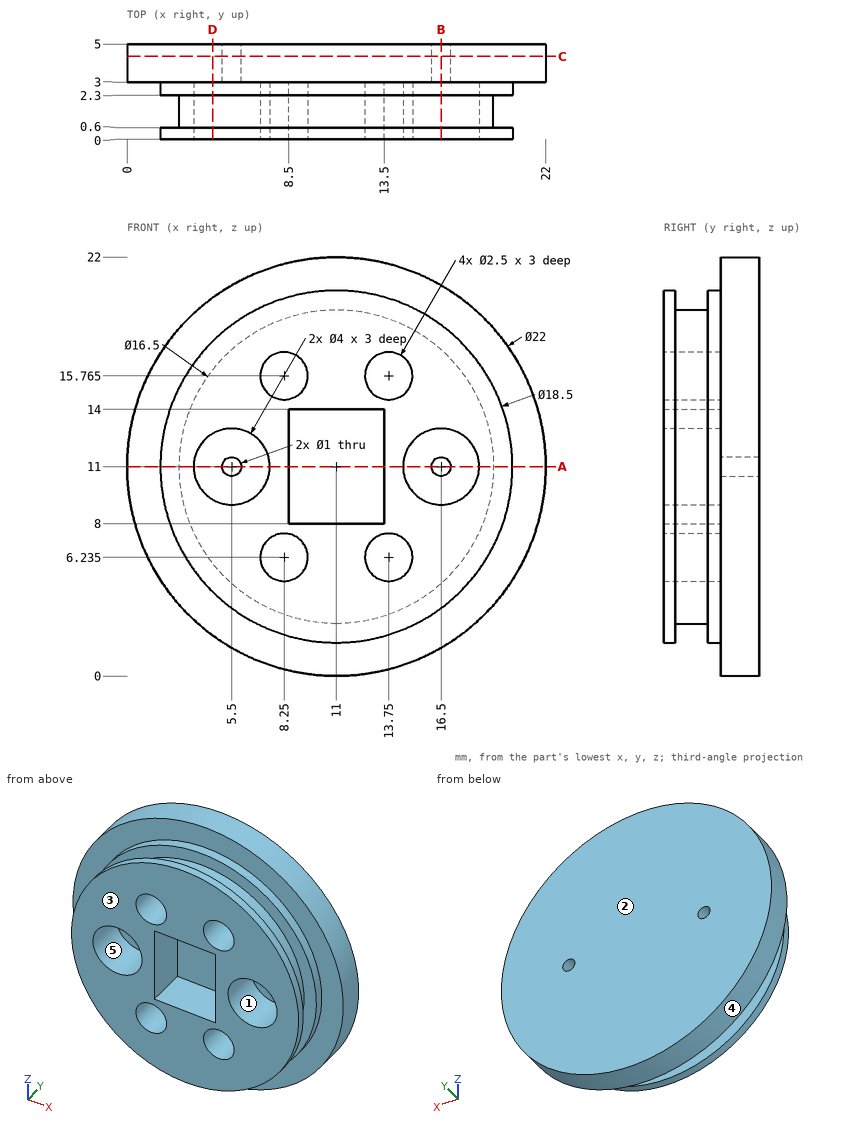
For this review, use the dimensioned drawing (mm, ordinates from the lowest corner) and the shaded views. A direction names the side the tool comes from. Coordinates: 2 decimals unless noted, no trailing zeros. Loops run counter-clockwise (first coordinate to the right, second up) from the corner with the lowest first, then second, coordinate; pieces in that order, holes last. Notation, with made-up numbers: (11.25, 23) -> (34.25, 23) arc R34 cw to (34.25, 54) -> close; hole circle Ø8 at (11.5, 46). An arc over 180 degrees is marked (long way). Write each question's results on one line, items separated by ' | '.
Q1. Mouldability with a two-part tool opening along Z and no side actions: class the marked faces 3, 4 and 5 as +Z half, -Z half, draft (parallel to the pull), parting line (faces both ways), or undercut.
Taken from the geometry:
face 3: draft | face 4: parting line | face 5: undercut
Q2. Machinability: for the marked faces 1 and 2, which of the approach directions +Z, -Z, +X, -X, +Y, -Y give a long, thin tool a straight path to every point of the face, cutting with its end or side? Answer none if there is none.
Taken from the geometry:
face 1: -Y | face 2: +Z, -Z, +X, -X, +Y
Q3. Add section B-B, the plane x = 16.5. State the section outline as (y, z) points, then the cut area to 3 significant figures.
Taken from the geometry:
outline: (0, 3.56) -> (0.6, 3.56) -> (0.6, 4.85) -> (2.3, 4.85) -> (2.3, 3.56) -> (3, 3.56) -> (3, 1.47) -> (5, 1.47) -> (5, 10.5) -> (3, 10.5) -> (3, 9) -> (0, 9) -> close; (0, 13) -> (3, 13) -> (3, 11.5) -> (5, 11.5) -> (5, 20.53) -> (3, 20.53) -> (3, 18.44) -> (2.3, 18.44) -> (2.3, 17.15) -> (0.6, 17.15) -> (0.6, 18.44) -> (0, 18.44) -> close | area: 64.3 mm²
Q4. Add section D-D, the plane x = 4.5. State the section outline as (y, z) points, then the cut area to 3 significant figures.
Taken from the geometry:
outline: (0, 4.42) -> (0.6, 4.42) -> (0.6, 5.92) -> (2.3, 5.92) -> (2.3, 4.42) -> (3, 4.42) -> (3, 2.13) -> (5, 2.13) -> (5, 19.87) -> (3, 19.87) -> (3, 17.58) -> (2.3, 17.58) -> (2.3, 16.08) -> (0.6, 16.08) -> (0.6, 17.58) -> (0, 17.58) -> (0, 12.73) -> (3, 12.73) -> (3, 9.27) -> (0, 9.27) -> close | area: 59.5 mm²
Q5. For pin 1 Ø1 at (x, y) = (18, 3) entering from +Z; pin 2 Ø2 at (x, z) = (16.5, 10.5) entering from -Y; pin 3 Ø9 at (x, z) = (8, 12) entering from -Y; pin 4 Ø1.5 at (x, y) = (10, 1.5) entering from -Z, all flat-tipped, find the tip position at first contact; note any pin that passes through.
Taken from the geometry:
pin 1: z = 19.87 | pin 2: y = 3 | pin 3: y = 0 | pin 4: z = 2.75
Q6. Add section A-A, the plane z = 11. Count the separate pieces of the cut face and the enclosed holes in it, then the cut area to 3 significant figures.
Taken from the geometry:
separate pieces: 3 | enclosed holes: 0 | area: 53.1 mm²
Q7. Add section C-C, the plane y = 4.35. State the section outline as (x, z) points, then the cut area to 3 significant figures.
Taken from the geometry:
outline: circle Ø22 at (11, 11); hole circle Ø1 at (5.5, 11); hole circle Ø1 at (16.5, 11) | area: 379 mm²
Q8. To check wall thickness, follow line 1 along X through (y, z) = (3.6, 11); line 2 along Z through (x, y) = (7.75, 0.8); line 3 along X through (y, z) = (2.05, 6.25). State the ranges of each line that lie inside material, in increasing order. Write a range as [from, to].
Taken from the geometry:
line 1: [0, 5], [6, 16], [17, 22] | line 2: [3.42, 5.09], [7.38, 14.62], [16.91, 18.58] | line 3: [4.25, 7], [9.5, 12.5], [15, 17.75]
